Source: CAD feature listing. Evaluate the final solid. Frame: model axes, mm. A direction names the side the tool comes from. Coordinates: 2 decimals unless noted, no trailing zeros. Loops run counter-clockwise (first coordinate to the right, second up) from the corner with the lowest first, then second, coordinate; pieces in that order, holes last. Notation, with made-up numbers: M -15,50.5 L 18,50.5 A18 cw 18,65.5 Z; hole C -7.5,45 d1. An arc over 180 degrees is marked long. One line per question, with ' | ' between items. Start each with the question number.
1. Section query B-B, the plane x = 0. Output: boundary loops of the cut face in (y, z) (3 decimals), and give its area (3 significant figures).
2. Section query C-C, the plane y = 0. Output: boundary loops of the cut face in (x, z) (3 decimals).
3. Section query D-D, the plane x = 7. Output: boundary loops of the cut face in (y, z).
4. Mould query, pull axis Y, two halves, no side actions, for faces 5 (the cylindrical face through (28, 0, 2)), 6 (the flat face through (13, -1, 4)), 7 (the flat face through (-2, 0, 3)), 8 (the flat face through (22, -3, 5)). Classes: pulls with the +Y half, pulls with the -Y half, needs draft (parallel to the pull), parting line crosses it, or undercut.
5. Pin query (flat end, axial travel): P1, Ø2.5, axis at x = 21, z = 5, coming from the -Y side; P2, Ø3.5, axis at x = 20, y = 0, coming from the -Z side; P3, Ø3.5, axis at x = 22, z = 5, coming from the +Y side; P4, Ø2.5, axis at x = 24, y = 0, coming from the -Z side. Return the tip coordinate at first contact, or that it passes through.
6. Ray query, probe 1 along Y at (x, z) = (24, 2.5); probe 2 along Y at (x, z) = (0, 2.3); probe 3 along Y at (x, z) = (22, 6). Return the intervals inside material, ascending.
7. Section query A-A, the plane z = 4.75. Output: boundary loops of the cut face in (x, y), and give its area (3 significant figures).
8. Access query for faces 1 (the flat face through (5, 0.5, 3)), 2 (the flat face through (0, -4, 6)), 3 (the cylindrical face through (27, 0, 5)), 4 (the flat face through (-5, 0.5, 5)). Directions: +Z, -Z, +X, -X, +Y, -Y. A direction counts if a zero-diameter tool reaches every point of the face in a straight line with its end or side. Return the directions, or none.
```python
from build123d import *

# Parameters (mm, degrees)
EXTRUDE_1_DEPTH     = 4
SKETCH_3_R          = 7.4
EXTRUDE_2_DEPTH     = 2
EXTRUDE_3_DEPTH     = 3
CUT_EXTRUDE_1_DEPTH = 3
SKETCH_7_R          = 1.5
CUT_EXTRUDE_2_DEPTH = 30.795301643
CUT_EXTRUDE_3_DEPTH = 30.795301643
SKETCH_10_R         = 3.925
CUT_EXTRUDE_4_DEPTH = 1.5


with BuildPart() as part:
    # ｽｹｯﾁ2 → ﾎﾞｽ - 押し出し1 (new body)
    with BuildSketch(Plane.XY):
        with BuildLine():
            Line((24, 4), (10.332473082, 4))
            ThreePointArc((10.332473082, 4), (7.206754774, 4.50105874), (4.394270162, 5.954022989))
            ThreePointArc((4.394270162, 5.954022989), (-7.4, 0), (4.394270162, -5.954022989))
            ThreePointArc((4.394270162, -5.954022989), (7.206754774, -4.50105874), (10.332473082, -4))
            Line((10.332473082, -4), (24, -4))
            ThreePointArc((24, -4), (28, 0), (24, 4))
        make_face()
    extrude(amount=EXTRUDE_1_DEPTH)

    # ｽｹｯﾁ3 → ﾎﾞｽ - 押し出し2 (add)
    with BuildSketch(Plane.XY.offset(4)):
        with Locations(Location((0, 0, 0), (0, 0, 53.571420986))):
            Circle(SKETCH_3_R)
    extrude(amount=EXTRUDE_2_DEPTH)

    # ｽｹｯﾁ4 → ﾎﾞｽ - 押し出し3 (add)
    with BuildSketch(Plane.XY.offset(4)):
        with BuildLine():
            Line((24, -3), (20, -3))
            ThreePointArc((20, -3), (17, 0), (20, 3))
            Line((20, 3), (24, 3))
            ThreePointArc((24, 3), (27, 0), (24, -3))
        make_face()
    extrude(amount=EXTRUDE_3_DEPTH)

    # ｽｹｯﾁ6 → ｶｯﾄ - 押し出し1 (cut)
    with BuildSketch(Plane.XY.offset(6)):
        with BuildLine():
            Line((7.4, 0.5), (2.958039892, 0.5))
            ThreePointArc((2.958039892, 0.5), (0, 3), (-2.958039892, 0.5))
            Line((-2.958039892, 0.5), (-7.4, 0.5))
            Line((-7.4, 0.5), (-7.4, -0.5))
            Line((-7.4, -0.5), (-2.958039892, -0.5))
            ThreePointArc((-2.958039892, -0.5), (0, -3), (2.958039892, -0.5))
            Line((2.958039892, -0.5), (7.4, -0.5))
            Line((7.4, -0.5), (7.4, 0.5))
        make_face()
    extrude(amount=-CUT_EXTRUDE_1_DEPTH, mode=Mode.SUBTRACT)

    # ｽｹｯﾁ7 → ｶｯﾄ - 押し出し2 (cut, through all)
    with BuildSketch(Plane.XY.offset(7)):
        with Locations((20, 0)):
            Circle(SKETCH_7_R)
        with Locations(Location((24, 0, 0), (0, 0, 180))):
            Circle(SKETCH_7_R)
    extrude(amount=-CUT_EXTRUDE_2_DEPTH, mode=Mode.SUBTRACT)

    # ｽｹｯﾁ8 → ｶｯﾄ - 押し出し3 (cut, through all)
    with BuildSketch(Plane(origin=(0, 0, 0), x_dir=(-1, 0, 0), z_dir=(0, 0, -1))):
        with BuildLine():
            ThreePointArc((-1.414213562, -0.5), (1.5, 0), (-1.414213562, 0.5))
            Line((-1.414213562, 0.5), (-7.495786438, 0.5))
            ThreePointArc((-7.495786438, 0.5), (-10.41, 0), (-7.495786438, -0.5))
            Line((-7.495786438, -0.5), (-1.414213562, -0.5))
        make_face()
    extrude(amount=-CUT_EXTRUDE_3_DEPTH, mode=Mode.SUBTRACT)

    # ｽｹｯﾁ10 → ｶｯﾄ - 押し出し4 (cut)
    with BuildSketch(Plane(origin=(0, 0, 0), x_dir=(-1, 0, 0), z_dir=(0, 0, -1))):
        Circle(SKETCH_10_R)
    extrude(amount=-CUT_EXTRUDE_4_DEPTH, mode=Mode.SUBTRACT)


solid = part.part
```
Taken from the geometry:
1) outline: M -7.4,0 L -3.925,0 L -3.925,1.5 L -1.5,1.5 L -1.5,3 L -3,3 L -3,6 L -7.4,6 Z; M 1.5,1.5 L 3.925,1.5 L 3.925,0 L 7.4,0 L 7.4,6 L 3,6 L 3,3 L 1.5,3 Z | area: 54.5 mm^2
2) outline: M -7.4,0 L -3.925,0 L -3.925,1.5 L -1.5,1.5 L -1.5,3 L -7.4,3 Z; M 10.41,0 L 18.5,0 L 18.5,7 L 17,7 L 17,4 L 10.41,4 Z; M 21.5,0 L 22.5,0 L 22.5,7 L 21.5,7 Z; M 25.5,0 L 28,0 L 28,4 L 27,4 L 27,7 L 25.5,7 Z
3) outline: M -4.57,0 L -0.5,0 L -0.5,6 L -2.4,6 L -2.4,4 L -4.57,4 Z; M 0.5,0 L 4.57,0 L 4.57,4 L 2.4,4 L 2.4,6 L 0.5,6 Z
4) face 5: parting line crosses it | face 6: needs draft | face 7: undercut | face 8: pulls with the -Y half
5) P1: y = -4 | P2: z = 0 | P3: y = 4 | P4: through
6) probe 1: -4 to -1.5, 1.5 to 4 | probe 2: -7.4 to -1.5, 1.5 to 7.4 | probe 3: -3 to 3
7) outline: M -7.38,-0.5 A7.4 ccw 7.38,-0.5 L 2.96,-0.5 A3 cw -2.96,-0.5 Z; M -7.38,0.5 L -2.96,0.5 A3 cw 2.96,0.5 L 7.38,0.5 A7.4 ccw Z; M 20,-3 L 24,-3 A3 ccw 24,3 L 20,3 A3 ccw Z; hole C 20,0 d3; hole C 24,0 d3 | area: 173 mm^2
8) face 1: +Z, -Z | face 2: +Z, -X, +Y, -Y | face 3: +Z, +X | face 4: +Z, -X
